Could you check a few things on this drawing? It's one solid part, dimensions in mm from its lowest x, y, z. Round coordinates to 2 decimals unless told otherwise and drop trailing zeros. Write each loop counter-clockwise with the first axis right and the second up, starting at its lowest first coordinate (ties: lowest second). Pieces come first, ordered by that corner, then holes. Notation, with made-up numbers: (37.25, 25) -> (74.25, 25) arc R4 cw to (74.25, 32) -> close; hole circle Ø8 at (-19, 41). An arc over 180 degrees is marked (long way). Return JSON: item names as keys, results as strings.
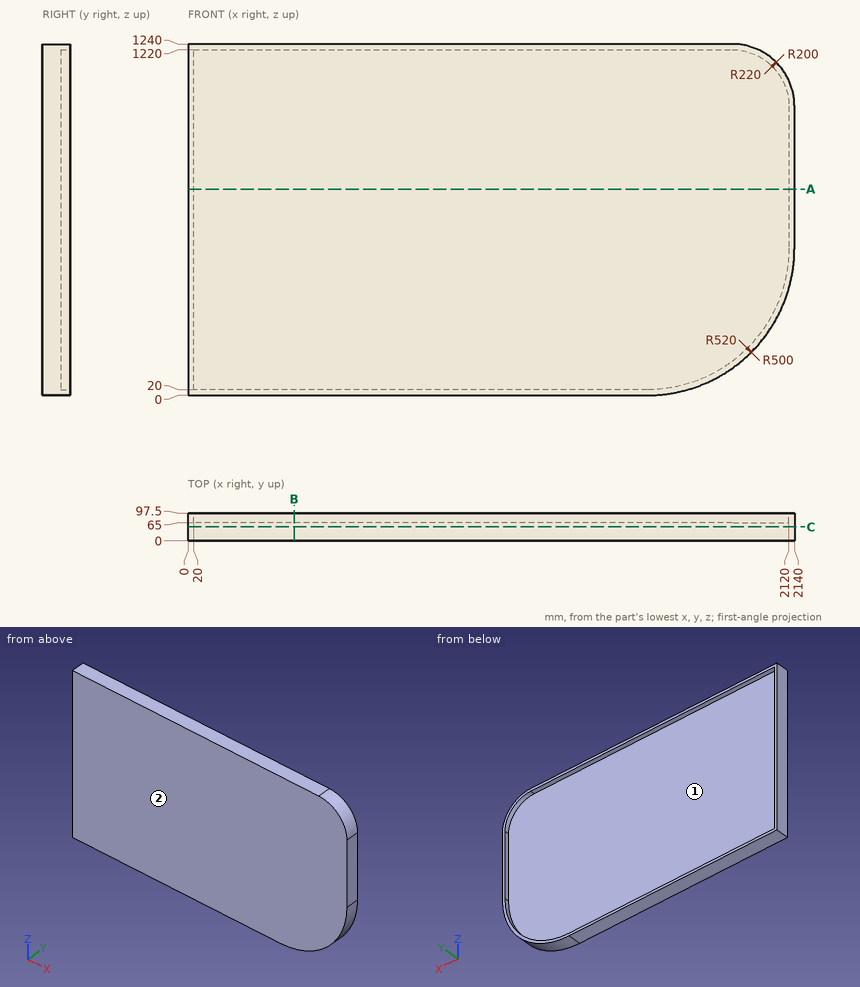
1) Thinking about a two-plate mould opening in X: for the marked faces 1 and 2, which applies, pulls with the +X half, pulls with the -X half, needs draft (parallel to the pull), parting line crosses it, or undercut?
Return value:
{"face 1": "undercut", "face 2": "needs draft"}
2) Will these pins go through, and if not, where does the flat tip stop? pin 1 Ø1.5 at (x, z) = (816, 854) entering from -Y; pin 2 Ø2 at (x, z) = (1644, 993.5) entering from +Y.
Return value:
{"pin 1": "y = 0", "pin 2": "y = 65"}
3) I want a section at A-A, the plane z = 728. Please give me the cut outline in (x, y).
Return value:
{"outline": "(0, 0) -> (2140, 0) -> (2140, 97.5) -> (2120, 97.5) -> (2120, 65) -> (20, 65) -> (20, 97.5) -> (0, 97.5) -> close"}
4) I want a section at C-C, the plane y = 50. Please give me the cut outline in (x, z).
Return value:
{"outline": "(0, 0) -> (1620, 0) arc R520 ccw to (2140, 520) -> (2140, 1020) arc R220 ccw to (1920, 1240) -> (0, 1240) -> close"}
5) I want a section at B-B, the plane x = 374. Please give me the cut outline in (y, z).
Return value:
{"outline": "(0, 0) -> (97.5, 0) -> (97.5, 20) -> (65, 20) -> (65, 1220) -> (97.5, 1220) -> (97.5, 1240) -> (0, 1240) -> close"}
6) If I drill on probe 1 along Z at (x, y) = (894, 91.5); probe 2 along Y at (x, z) = (1923.5, 513); probe 3 along X at (y, z) = (91, 1015.5), over which ranges is the centre line in solid material (lowest first)? Write a range as [from, to].
Return value:
{"probe 1": "[0, 20], [1220, 1240]", "probe 2": "[0, 65]", "probe 3": "[0, 20], [2120, 2140]"}
